from build123d import *

# Parameters (mm, degrees)
BASE_FLANGE2_DEPTH                                 = 825.5
SKETCH1_R                                          = 3.175
SKETCH1_R_2                                        = 2.413
SKETCH1_R_3                                        = 5.55625
SKETCH1_R_4                                        = 2.5527
SKETCH1_R_5                                        = 2.0447
SKETCH1_R_6                                        = 14.28115
SKETCH1_R_7                                        = 11.10615
SKETCH1_R_8                                        = 1.5875
SKETCH1_R_9                                        = 9.525
SKETCH1_R_10                                       = 1.27
SKETCH1_R_11                                       = 34.925
CUT_EXTRUDE3_DEPTH                                 = 859.694710551
CSK_FOR_10_FLAT_HEAD_MACHINE_SCREW_100_D           = 4.9784
CSK_FOR_10_FLAT_HEAD_MACHINE_SCREW_100_CSINK_D     = 9.779
CSK_FOR_10_FLAT_HEAD_MACHINE_SCREW_100_CSINK_ANGLE = 100
SKETCH8_R                                          = 0.635
CUT_EXTRUDE4_DEPTH                                 = 860.130662682
F_1_4_CLEARANCE_HOLE1_D                            = 6.5278
F_1_4_CLEARANCE_HOLE1_DEPTH                        = 1.5875
F_8_CLEARANCE_HOLE1_D                              = 4.9149
F_8_CLEARANCE_HOLE1_DEPTH                          = 1.5875


# Sheet-metal steps are written as plain solids
with BuildPart() as part:
    # Sketch3 → Base-Flange2 (new body)
    with BuildSketch(Plane.XY):
        with BuildLine():
            Line((3.175, 233.4895), (25.4, 233.4895))
            Line((25.4, 233.4895), (25.4, 235.077))
            Line((25.4, 235.077), (3.175, 235.077))
            ThreePointArc((3.175, 235.077), (0.92993597, 234.14706403), (0, 231.902))
            Line((0, 231.902), (0, 0))
            ThreePointArc((0, 0), (0.92993597, -2.24506403), (3.175, -3.175))
            Line((3.175, -3.175), (25.4, -3.175))
            Line((25.4, -3.175), (25.4, -1.5875))
            Line((25.4, -1.5875), (3.175, -1.5875))
            ThreePointArc((3.175, -1.5875), (2.052467985, -1.122532015), (1.5875, 0))
            Line((1.5875, 0), (1.5875, 231.902))
            ThreePointArc((1.5875, 231.902), (2.052467985, 233.024532015), (3.175, 233.4895))
        make_face()
    extrude(amount=-BASE_FLANGE2_DEPTH)

    # Sketch1 → Cut-Extrude3 (cut, through all)
    with BuildSketch(Plane(origin=(0, 0, 0), x_dir=(0, 0, -1), z_dir=(1, 0, 0))):
        with Locations(Location((516.509, 31.75, 0), (0, 0, 90))):
            Circle(SKETCH1_R)
        with Locations(Location((308.991, 31.75, 0), (0, 0, 90))):
            Circle(SKETCH1_R)
        with Locations(Location((103.492550911, 60.630923565, 0), (0, 0, 90))):
            Circle(SKETCH1_R)
        with Locations(Location((722.007449089, 60.630923565, 0), (0, 0, 90))):
            Circle(SKETCH1_R)
        with Locations(Location((412.75, 6.35, 0), (0, 0, 90))):
            Circle(SKETCH1_R_2)
        with Locations(Location((412.75, 88.9, 0), (0, 0, 90))):
            Circle(SKETCH1_R_2)
        with Locations(Location((622.478249316, 6.35, 0), (0, 0, 90))):
            Circle(SKETCH1_R_2)
        with Locations(Location((612.465522577, 88.9, 0), (0, 0, 90))):
            Circle(SKETCH1_R_2)
        with Locations(Location((203.021750684, 6.35, 0), (0, 0, 90))):
            Circle(SKETCH1_R_2)
        with Locations(Location((101.978503418, 46.225723918, 0), (0, 0, 90))):
            Circle(SKETCH1_R)
        with Locations(Location((723.521496582, 46.225723918, 0), (0, 0, 90))):
            Circle(SKETCH1_R)
        with Locations(Location((213.034477423, 88.9, 0), (0, 0, 90))):
            Circle(SKETCH1_R_2)
        with Locations(Location((466.319936913, 184.736959746, 0), (0, 0, 90))):
            Circle(SKETCH1_R_3)
        with Locations(Location((483.337936913, 177.751959746, 0), (0, 0, 90))):
            Circle(SKETCH1_R_4)
        with Locations(Location((483.337936913, 183.593959746, 0), (0, 0, 90))):
            Circle(SKETCH1_R_5)
        with Locations(Location((483.337936913, 114.251959746, 0), (0, 0, 90))):
            Circle(SKETCH1_R_4)
        with Locations(Location((483.337936913, 108.409959746, 0), (0, 0, 90))):
            Circle(SKETCH1_R_5)
        with Locations(Location((466.319936913, 107.266959746, 0), (0, 0, 90))):
            Circle(SKETCH1_R_3)
        with Locations(Location((440.919936913, 107.266959746, 0), (0, 0, 90))):
            Circle(SKETCH1_R_3)
        with Locations(Location((415.519936913, 107.266959746, 0), (0, 0, 90))):
            Circle(SKETCH1_R_3)
        with Locations(Location((394.437936913, 107.266959746, 0), (0, 0, 90))):
            Circle(SKETCH1_R_4)
        with Locations(Location((394.437936913, 101.424959746, 0), (0, 0, 90))):
            Circle(SKETCH1_R_5)
        with Locations(Location((394.437936913, 184.736959746, 0), (0, 0, 90))):
            Circle(SKETCH1_R_4)
        with Locations(Location((394.437936913, 190.578959746, 0), (0, 0, 90))):
            Circle(SKETCH1_R_5)
        with Locations(Location((412.75, 146.001959746, 0), (0, 0, 90))):
            Circle(SKETCH1_R_6)
        with Locations(Location((453.4662, 146.001959746, 0), (0, 0, 90))):
            Circle(SKETCH1_R_7)
        with Locations(Location((440.919936913, 184.736959746, 0), (0, 0, 90))):
            Circle(SKETCH1_R_3)
        with Locations(Location((415.519936913, 184.736959746, 0), (0, 0, 90))):
            Circle(SKETCH1_R_3)
        with Locations(Location((345.35745, 97.70745, 0), (0, 0, 90))):
            Circle(SKETCH1_R_8)
        with Locations(Location((315.04255, 97.70745, 0), (0, 0, 90))):
            Circle(SKETCH1_R_8)
        with Locations(Location((315.04255, 67.39255, 0), (0, 0, 90))):
            Circle(SKETCH1_R_8)
        with Locations(Location((345.35745, 67.39255, 0), (0, 0, 90))):
            Circle(SKETCH1_R_8)
        with Locations(Location((330.2, 82.55, 0), (0, 0, 90))):
            Circle(SKETCH1_R_9)
        with Locations(Location((361.95, 211.6836, 0), (0, 0, 90))):
            Circle(SKETCH1_R_10)
        with Locations(Location((298.45, 211.6836, 0), (0, 0, 90))):
            Circle(SKETCH1_R_10)
        with Locations(Location((298.45, 148.1836, 0), (0, 0, 90))):
            Circle(SKETCH1_R_10)
        with Locations(Location((361.95, 148.1836, 0), (0, 0, 90))):
            Circle(SKETCH1_R_10)
        with Locations(Location((330.2, 179.9336, 0), (0, 0, 90))):
            Circle(SKETCH1_R_11)
        Polygon((825.5, -3.175), (775.673017562, -3.175), (825.5, 107.95), align=None)
        Polygon((0, 107.95), (0, -3.175), (49.826982438, -3.175), align=None)
    extrude(amount=CUT_EXTRUDE3_DEPTH, mode=Mode.SUBTRACT)

    # CSK for #10 Flat Head Machine Screw (100)1 (through all)
    with Locations(Plane.ZY):
        with Locations((-345.35745, 97.70745), (-315.04255, 97.70745), (-315.04255, 67.39255), (-345.35745, 67.39255), (-298.45, 148.1836), (-361.95, 148.1836), (-361.95, 211.6836), (-298.45, 211.6836)):
            CounterSinkHole(CSK_FOR_10_FLAT_HEAD_MACHINE_SCREW_100_D / 2, CSK_FOR_10_FLAT_HEAD_MACHINE_SCREW_100_CSINK_D / 2, counter_sink_angle=CSK_FOR_10_FLAT_HEAD_MACHINE_SCREW_100_CSINK_ANGLE)

    # Sketch8 → Cut-Extrude4 (cut, through all)
    with BuildSketch(Plane(origin=(0, -1.5875, 0), x_dir=(1, 0, 0), z_dir=(0, 1, 0))):
        with Locations(Location((14.2875, 382.481016783, 0), (0, 0, 180))):
            Circle(SKETCH8_R)
        with Locations(Location((14.2875, 369.781016783, 0), (0, 0, 180))):
            Circle(SKETCH8_R)
        with Locations(Location((14.2875, 357.081016783, 0), (0, 0, 180))):
            Circle(SKETCH8_R)
        with Locations(Location((14.2875, 344.381016783, 0), (0, 0, 180))):
            Circle(SKETCH8_R)
        with Locations(Location((14.2875, 331.681016783, 0), (0, 0, 180))):
            Circle(SKETCH8_R)
        with Locations(Location((14.2875, 318.981016783, 0), (0, 0, 180))):
            Circle(SKETCH8_R)
        with Locations(Location((14.2875, 306.281016783, 0), (0, 0, 180))):
            Circle(SKETCH8_R)
        with Locations(Location((14.2875, 293.581016783, 0), (0, 0, 180))):
            Circle(SKETCH8_R)
    extrude(amount=-CUT_EXTRUDE4_DEPTH, mode=Mode.SUBTRACT)

    # 1/4 Clearance Hole1
    with Locations(Plane(origin=(0, -1.5875, 0), x_dir=(1, 0, 0), z_dir=(0, 1, 0))):
        with Locations((14.2875, 382.481016783), (14.2875, 369.781016783), (14.2875, 357.081016783), (14.2875, 344.381016783), (14.2875, 331.681016783), (14.2875, 318.981016783), (14.2875, 306.281016783), (14.2875, 293.581016783)):
            Hole(F_1_4_CLEARANCE_HOLE1_D / 2, depth=F_1_4_CLEARANCE_HOLE1_DEPTH)

    # #8 Clearance Hole1
    with Locations(Plane(origin=(0, 233.4895, 0), x_dir=(-1, 0, 0), z_dir=(0, -1, 0))):
        with Locations((-14.2875, 279.4), (-14.2875, 266.7), (-14.2875, 254), (-14.2875, 241.3), (-14.2875, 228.6), (-14.2875, 215.9), (-14.2875, 203.2), (-14.2875, 190.5)):
            Hole(F_8_CLEARANCE_HOLE1_D / 2, depth=F_8_CLEARANCE_HOLE1_DEPTH)


solid = part.part
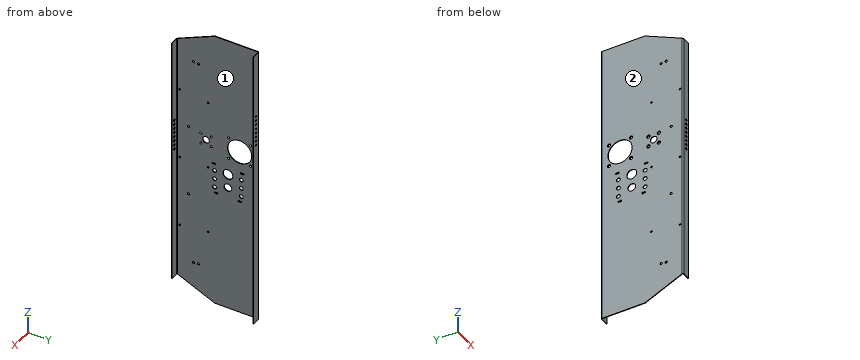
CAD build for the part. Positions are in the model's coordinates, mm. Face numbers are marked on the shaded views. Round coordinates to 2 decimals unless told otherwise and drop trailing zeros. Use one line per item in the form item = value.
Q1. Flat gauge pins, fed straight in: P1, Ø8.5, axis at y = 60.63, z = -722.01, coming from the +X side; P2, Ø9, axis at y = 107.27, z = -440.92, coming from the +X side; P3, Ø4.5, axis at x = 14.29, z = -279.4, coming from the +Y side. Where does each tip first touch, or does it go through?
Recorded:
P1 = 1.59
P2 = through
P3 = -1.59
Q2. Probe L1, parallel to Y at x = 14.75, z = -591 (1 decimal); L2, parallel to Z at x = 0.8, y = 88.9; L3, parallel to X at y = 172, z = -628.5. List the from-to ranges inside material, lowest first.
Recorded:
L1 = -3.2 to -1.6, 233.5 to 235.1
L2 = -816.96 to -614.88, -610.05 to -415.16, -410.34 to -337.3, -323.1 to -215.45, -210.62 to -8.54
L3 = 0 to 1.59
Q3. Two-plate mould, pull along Y, no slides. Class the marked faces 1 and 2: +Y half, -Y half, draft (parallel to the pull), parting line (faces both ways), or undercut.
Recorded:
face_1 = undercut
face_2 = draft
